Model file for the job. Use its own axes, mm. Give positions to 0.01 mm unless a question says otherwise; leave off trailing zeros. Loops run counter-clockwise (first coordinate to the right, second up) from the corner with the lowest first, then second, coordinate; pieces in that order, holes last. Notation, with made-up numbers: M 41.25,62 L 55.25,62 A6 cw 55.25,66 Z; hole C 13.25,-10.75 d6. An arc over 180 degrees is marked long. Answer in a Markdown table with one row per item.
Autodesk Inventor part; units mm, degrees
ref_plane "Zahnebene" through (0, -10, 0) normal (-0.2940858, 0, 0.955779) x (0, 1, 0)
ref_plane "Work Plane13" through (0, 0, 0) normal (-0.309017, 0.9510565, 0) x (0, 0, 1)
ref_plane "Work Plane14" through (0, 0, 0) normal (0.9510565, 0.309017, 0) x (0, 0, 1)
ref_plane "Zahnebene" through (0, -10, 0) normal (-0.2940858, 0, 0.955779) x (0, 1, 0)
sketch "Grundkörperskizze" plane through (0, 0, 0) normal (1, 0, 0) x (0, 1, 0)
  line L0 (0, -5.95) -> (0, 5.95)
  line L1 (0, 2.5) -> (3.9106, 2.5)
  line L2 (3.9106, 2.5) -> (5.525, 1.8118)
  line L3 (-2.72, 0) -> (16.32, 0) construction
  circle A0 centre (9.775, 0) radius 4.675
  line L4 (5.525, 1.8118) -> (5.525, -1.8118)
  line L5 (0, -2.5) -> (3.9106, -2.5)
  line L6 (0, 2.5) -> (0, -2.5)
  line L7 (3.9106, -2.5) -> (5.525, -1.8118)
  dimension "d50" = 23.089
  dimension "d87" = 11.05
  dimension "d89" = 9.35
  dimension "d92" = 5
  dimension "d93" = 9.775
revolve "Grundkörper" add sketch "Grundkörperskizze" angle 360 about axis through (0, 0, 0) along (0, 0, 1) picked at (5.4149, 0.3119) contours L0 L1 L2 A0 L7 L5 | A0 L2 L4 L7
revolve "Grundkörper2" cut sketch "Grundkörperskizze" angle 360 about axis through (0, 0, 0) along (0, 0, 1) contours L7 L4 L2 A0 | A0 L2 L4 L7
sketch "Zahnskizze" plane through (0, -10, 0) normal (-0.2940858, 0, 0.955779) x (0, 1, 0)
  line L0 (10, 1.6413) -> (10, -1.6413)
  line L1 (-0.574, 0) -> (7.994, 0)
  line L2 (0.225, 1.1724) -> (0.225, -1.1724)
  line L3 (0.225, -1.1724) -> (4.73, -1.1724)
  line L4 (4.73, -1.1724) -> (6.77, -0.4299)
  line L5 (6.77, -0.4299) -> (6.77, 0)
  line L6 (6.77, 0.4299) -> (4.73, 1.1724)
  line L7 (4.73, 1.1724) -> (0.225, 1.1724)
  line L8 (6.77, 0.4299) -> (6.77, 0)
  line L9 (5.75, 0) -> (5.75, -0.8011) construction
  dimension "d38" = 9.775
  dimension "d39" = 20
  dimension "d40" = 4.505
  dimension "d41" = 5.525
  dimension "d42" = 0.8011
sketch "Sketch8" plane through (0, 0, 2.5) normal (0, 0, 1) x (1, 0, 0)
  circle A0 centre (0, 0) radius 3.9106
  circle A1 centre (0, 0) radius 4.25
  dimension "d77" = 8.5
surface extrude "Flankendurchmesser" sketch "Sketch8" against normal blind 5 shown no curves A1
ref_plane "Work Plane13" through (0, 0, 0) normal (-0.309017, 0.9510565, 0) x (0, 0, 1)
revolve "Zahn" [suppressed]
pattern_circular "Zahnanordnung" [suppressed]
ref_plane "Work Plane14" through (0, 0, 0) normal (0.9510565, 0.309017, 0) x (0, 0, 1)
ref_plane "Work Plane15" through (0, 0, 0) normal (0, -1, 0) x (0, 0, 1)
equation "\"d50\" = da_fi"
equation "\"d87\" = da_dae"
equation "\"d89\" = 2 * da_aw - da_da"
equation "\"d92\" = da_b"
equation "\"d93\" = da_aw"
equation "\"d38\" = da_aw"
equation "\"d39\" = da_alfat"
equation "\"d40\" = 0.5 * da_df1"
equation "\"d41\" = 0.5 * da_d1"
equation "\"d42\" = 0.3 * da_px"
equation "\"d77\" = da_dw"
equation "\"d78\" = da_b"
equation "\"da_aw\" = 9.775"
equation "\"da_fi\" = 23.0888deg"
equation "\"da_b\" = 5"
equation "\"da_df\" = 6.46"
equation "\"da_da\" = 10.2"
equation "\"da_beta\" = 17.102729deg"
equation "\"da_alfat\" = 20deg"
equation "\"da_df1\" = 9.01"
equation "\"da_da1\" = 12.75"
equation "\"da_d1\" = 11.05"
equation "\"da_px\" = 2.67035"
equation "\"d68\" = da_aw"
equation "\"da_dw\" = 8.5"
equation "\"da_rightdir\" = 0"
equation "\"d86\" = da_aw"
equation "\"da_dae\" = 11.05"
properties part number "Schneckenrad" material "Steel, Mild"
(1) Wall check: L1, parallel to Y at x = -1.75, z = -1.2; L2, parallel to X at y = -2, z = -0.75; L3, parallel to X at y = -4.25, z = -1.7. Give the ranges that are in metal, low to high.
Established:
| item | result |
|---|---|
| L1 | y = -4.96 to 4.96 |
| L2 | x = -4.76 to 4.76 |
| L3 | x = -3.36 to 3.36 |
(2) Saw through at C-C, the plane z = -2.05. Give the cut face in (x, y), and give its area (3 significant figures).
Established:
| item | result |
|---|---|
| outline | C 0,0 d9.93 |
| area | 77.5 mm2 |
(3) Saw through at D-D, the plane z = 1.5. Give the cut face in (x, y), and give its area (3 significant figures).
Established:
| item | result |
|---|---|
| outline | C 0,0 d10.69 |
| area | 89.8 mm2 |
(4) Flat gauge pin, fed straight in: P1, Ø1, axis at x = -3.5, y = 4, coming from the +Z side. Where does the tip first touch, or does it go through?
Established:
| item | result |
|---|---|
| P1 | stops at z = 2.11 |
(5) Saw through at A-A, the plane y = 0. Give the cut face in (x, z) (3 decimals), and give its area (3 significant figures).
Established:
| item | result |
|---|---|
| outline | M -5.474,-1.833 L -3.911,-2.5 L 3.911,-2.5 L 5.474,-1.833 A4.675 cw 5.474,1.833 L 3.911,2.5 L -3.911,2.5 L -5.474,1.833 A4.675 cw Z |
| area | 50.8 mm2 |
